from build123d import *

# Parameters (mm, degrees)
F1_DEPTH = 2.54
F2_R     = 12.5
F3_DEPTH = 25.4


with BuildPart() as f1:
    # F0 (on Top) → F1 (new body)
    with BuildSketch(Plane.XY):
        with BuildLine():
            ThreePointArc((98.582891, 38.180412), (55.952119, 99.644459), (0, 50))
            ThreePointArc((0, 50), (-55.952119, 99.644459), (-98.582891, 38.180412))
            Line((-98.582891, 38.180412), (-56.351205, 0.405018))
            Line((-56.351205, 0.405018), (0, -50))
            Line((0, -50), (56.351205, 0.405018))
            Line((56.351205, 0.405018), (98.582891, 38.180412))
        make_face()
    extrude(amount=F1_DEPTH)

    # F2 (on face) → F3 (cut)
    with BuildSketch(Plane.XY.offset(2.54)):
        with Locations((0, 35)):
            Circle(F2_R)
    extrude(amount=-F3_DEPTH, mode=Mode.SUBTRACT)


solid = f1.part
For this review, take the finished solid that the model builds, in its own axes (mm). Round coordinates to 2 decimals unless told otherwise and drop trailing zeros. Loops run counter-clockwise (first coordinate to the right, second up) from the corner with the lowest first, then second, coordinate; pieces in that order, holes last. Notation, with made-up numbers: (44.5, -9.5) - (99.5, -9.5) arc R29 cw to (99.5, 19.5) - close; hole circle Ø7 at (0.25, 49.25). An arc over 180 degrees is marked (long way). One line per item, written item: value. Start each with the question number.
Item 1: Take a section at C-C (y = 35). Give the boundary of the cut face in (x, z), plus the area to 3 significant figures.
Item 2: For L1, parallel to X at y = 76, z = 1; L2, parallel to X at y = 59, z = 2.1; L3, parallel to X at y = 3.5, z = 0.55, list the stretches that pass through material, from the lowest coordinate up.
Item 3: The part is to be moulded in two halves that separate along X. For faces 1 (the flat face through (-1, 59, 2.54)), 2 (the cylindrical face through (-2.71, 22.797, 1.288)), say which applies: +X half, -X half, draft (parallel to the pull), parting line (faces both ways), or undercut.
Item 4: Take a section at A-A (y = 80). Give the boundary of the cut face in (x, z).
Item 5: Take a section at B-B (z = 1.6). Give the boundary of the cut face in (x, y).
Item 6: Take a section at D-D (x = -58.5). Give the boundary of the cut face in (y, z).
Item 7: Clearance check with flat-ended pins moving along their axes: pin 1 Ø1 at (y, z) = (-30.5, 1.5) entering from +X; pin 2 Ø22.5 at (x, y) = (0, 35) entering from -Z; pin 3 Ø1 at (x, z) = (63, 1) entering from -Y (3 decimals). State where each tip first meets the part, or that it passes through.
Answer below:
1. outline: (-95.03, 0) - (-12.5, 0) - (-12.5, 2.54) - (-95.03, 2.54) - close; (12.5, 0) - (95.03, 0) - (95.03, 2.54) - (12.5, 2.54) - close
1. area: 419 mm2
2. L1: x = -92.71 to -7.29, 7.29 to 92.71
2. L2: x = -99.18 to -0.82, 0.82 to 99.18
2. L3: x = -59.81 to 59.81
3. face 1: draft
3. face 2: undercut
4. outline: (-90, 0) - (-10, 0) - (-10, 2.54) - (-90, 2.54) - close; (10, 0) - (90, 0) - (90, 2.54) - (10, 2.54) - close
5. outline: (-98.58, 38.18) - (0, -50) - (98.58, 38.18) arc R50 ccw (long way) to (0, 50) arc R50 ccw (long way) to start; hole circle Ø25 at (0, 35)
6. outline: (2.33, 0) - (99.27, 0) - (99.27, 2.54) - (2.33, 2.54) - close
7. pin 1: stops at x = 22.36
7. pin 2: passes through
7. pin 3: stops at y = 5.905
